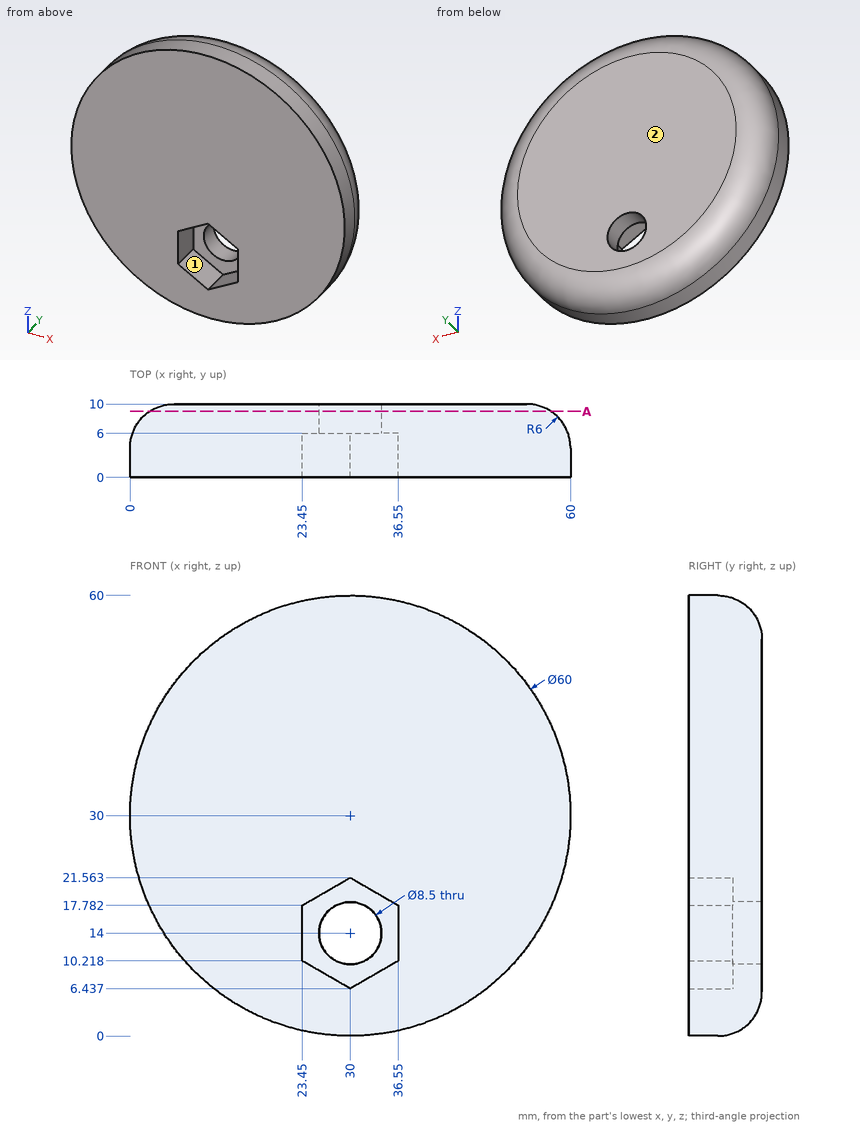
Geometry: see drawing. Coordinates: mm, zero at the bounding-box minimum. A direction names the side the tool comes from. Give positions to 0.01 mm unless a question says otherwise; leave off trailing zeros. Loops run counter-clockwise (first coordinate to the right, second up) from the corner with the lowest first, then second, coordinate; pieces in that order, holes last. Notation, with made-up numbers: (11, 50) - (56, 50) arc R21 ccw to (56, 71) - close; hole circle Ø11 at (15.5, 71). An arc over 180 degrees is marked (long way). One line per question, with ' | ' between items. Start each with the question number.
(1) Reachability of the marked faces 1 and 2 from +Z, -Z, +X, -X, +Y, -Y: full face, straight path, thin tool, end or side. Return the list, or none.
(2) Contact query for flat-ended pins moving along their axis: pin 1 (5 mm diameter, centred on y = 4, z = 13, fed in from -X); pin 2 (4 mm diameter, centred on x = 7.5, y = 5, fed in from +Z) (1 decimal); pin 3 (5 mm diameter, centred on y = 1.5, z = 15.5, fed in from +X) (1 decimal). Output: stop coordinate, or through.
(3) Section query A-A on y = 9. Return loops of the section in (x, z).
(4) Ray query, line 1 (Z direction, x = 30, y = 7.6); line 2 (Z direction, x = 30, y = 7.05); line 3 (X direction, y = 5.5, z = 49). Return the intervals inside material, ascending. Write a range as from..to.
The answers:
1) face 1: -Y | face 2: +Z, -Z, +X, -X, +Y
2) pin 1: x = 3.74 | pin 2: z = 51.8 | pin 3: x = 57.5
3) outline: circle Ø54.63 at (30, 30); hole circle Ø8.5 at (30, 14)
4) line 1: 1.2..9.75, 18.25..58.8 | line 2: 0.83..9.75, 18.25..59.17 | line 3: 7.03..52.97
